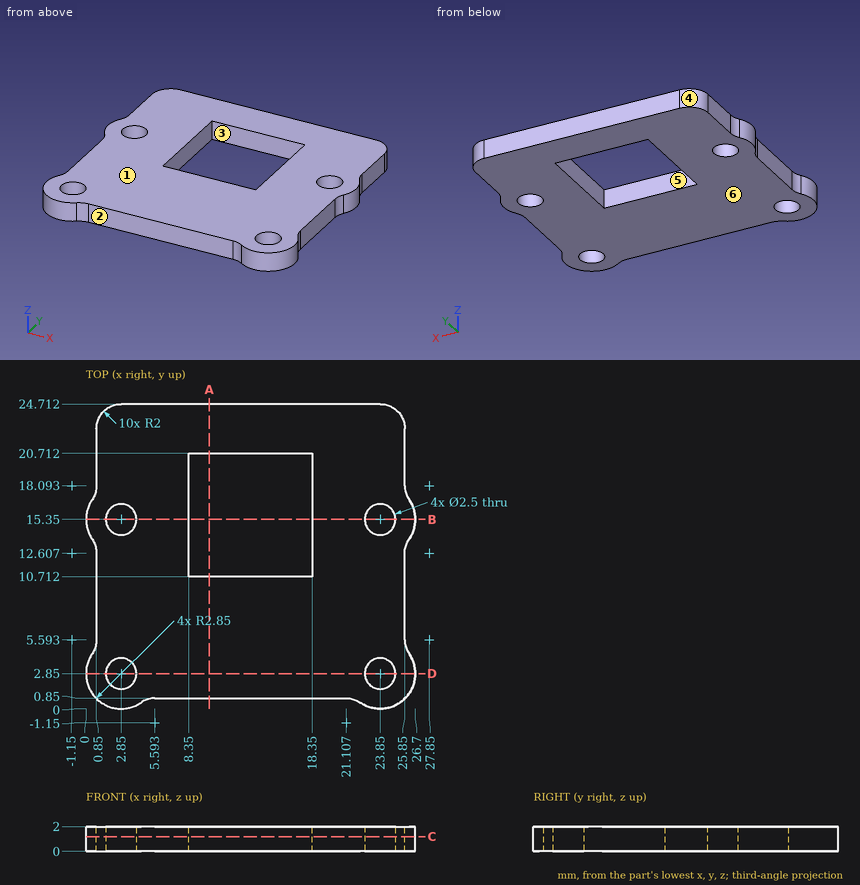
Input: dimensioned drawing with shaded views. Units: mm. Origin: part minimum x, y, z. A direction names the side the tool comes from. Give positions to 0.01 mm unless a question says otherwise; leave off trailing zeros. Loops run counter-clockwise (first coordinate to the right, second up) from the corner with the lowest first, then second, coordinate; pieces in that order, holes last. Notation, with made-up numbers: (3.25, 83) - (17.25, 83) arc R16 cw to (17.25, 99) - close; hole circle Ø1 at (89, 57). An arc over 180 degrees is marked (long way). Answer as CSV lines item,"result". Start each with the question number.
(1) Section query A-A (x = 10). Output: boundary loops of the cut face in (y, z), and give its area (3 significant figures).
(2) Ray query, line 1 along Y through (x, z) = (23.85, 1.4); line 2 along Y through (x, z) = (2.25, 0.2) (1 decimal); line 3 along Y through (x, z) = (13.25, 0.65). Return the intervals inside material, ascending. Write a range as [from, to].
(3) Section query C-C (z = 1.2). Output: boundary loops of the cut face in (x, y), and give its area (3 significant figures).
(4) Section query B-B (y = 15.35). Output: boundary loops of the cut face in (x, z).
(5) Reachability of the marked faces 1, 2 and 3 from +Z, -Z, +X, -X, +Y, -Y: full face, straight path, thin tool, end or side. Return the list, or none.
(6) Section query D-D (y = 2.85). Output: boundary loops of the cut face in (x, z).
(7) Mould query, pull axis X, two halves, no side actions, for the marked faces 4, 5 and 6. Classes: +X half, -X half, draft (parallel to the pull), parting line (faces both ways), or undercut.
(8) Pin query (flat end, axial travel): P1, Ø0.6, axis at y = 8, z = 1, coming from the +X side; P2, Ø1, axis at y = 10, z = 1, coming from the -X side; P3, Ø1, axis at x = 11.5, z = 1.5, coming from the -Y side. Return the tip coordinate at first contact, or that it passes through.
Worked answers:
1,outline,"(0.85, 0) - (10.71, 0) - (10.71, 2) - (0.85, 2) - close; (20.71, 0) - (24.71, 0) - (24.71, 2) - (20.71, 2) - close"
1,area,"27.7 mm^2"
2,line 1,"y = [0, 1.6], [4.1, 14.1], [16.6, 24.71]"
2,line 2,"y = [0.1, 1.8], [3.9, 14.3], [16.4, 24.6]"
2,line 3,"y = [0.85, 10.71], [20.71, 24.71]"
3,outline,"(0.5, 4.46) arc R2.85 ccw to (4.46, 0.5) arc R2 cw to (5.59, 0.85) - (21.11, 0.85) arc R2 cw to (22.24, 0.5) arc R2.85 ccw to (26.2, 4.46) arc R2 cw to (25.85, 5.59) - (25.85, 12.61) arc R2 cw to (26.2, 13.74) arc R2.85 ccw to (26.2, 16.96) arc R2 cw to (25.85, 18.09) - (25.85, 22.71) arc R2 ccw to (23.85, 24.71) - (2.85, 24.71) arc R2 ccw to (0.85, 22.71) - (0.85, 18.09) arc R2 cw to (0.5, 16.96) arc R2.85 ccw to (0.5, 13.74) arc R2 cw to (0.85, 12.61) - (0.85, 5.59) arc R2 cw to start; hole circle Ø2.5 at (2.85, 2.85); hole circle Ø2.5 at (2.85, 15.35); hole (8.35, 10.71) - (18.35, 10.71) - (18.35, 20.71) - (8.35, 20.71) - close; hole circle Ø2.5 at (23.85, 2.85); hole circle Ø2.5 at (23.85, 15.35)"
3,area,"490 mm^2"
4,outline,"(0, 0) - (1.6, 0) - (1.6, 2) - (0, 2) - close; (4.1, 0) - (8.35, 0) - (8.35, 2) - (4.1, 2) - close; (18.35, 0) - (22.6, 0) - (22.6, 2) - (18.35, 2) - close; (25.1, 0) - (26.7, 0) - (26.7, 2) - (25.1, 2) - close"
5,face 1,"+Z, +X, -X, +Y, -Y"
5,face 2,"+Z, -Z, -Y"
5,face 3,"+Z, -Z"
6,outline,"(0, 0) - (1.6, 0) - (1.6, 2) - (0, 2) - close; (4.1, 0) - (22.6, 0) - (22.6, 2) - (4.1, 2) - close; (25.1, 0) - (26.7, 0) - (26.7, 2) - (25.1, 2) - close"
7,face 4,"-X half"
7,face 5,"undercut"
7,face 6,"draft"
8,P1,"stops at x = 25.85"
8,P2,"stops at x = 0.85"
8,P3,"stops at y = 0.85"
